Can you work these out from the model? Positions are in its coordinate system, mm. Give positions to 0.01 mm unless a question says otherwise; leave off trailing zeros. Order: outer loops, then holes, each group sorted by start corner. A loop starts at its lowest first (then second) coordinate and runs counter-clockwise, first axis right, second up. Notation, with made-up numbers: M -37,61 L -2,61 A20 ccw -2,94 Z; hole C 65,18.5 d8. An arc over 180 degrees is marked long. Write each question's results on one line, items separated by ' | '.
Solid Edge part; units mm, degrees
sketch "Sketch1" plane through (0, 0, 0) normal (-1, 0, 0) x (0, -1, 0)
  line L0 (0, 20) -> (-5, 20)
  line L1 (-5, 20) -> (-5, 0)
  line L2 (-5, 0) -> (0, 0)
  line L3 (0, 0) -> (0, 20)
extrude "Protrusion1" add sketch "Sketch1" along normal mid plane 90
sketch "Sketch2" plane through (0, 0, 7.5) normal (0, -1, 0) x (1, 0, 0)
  line L0 (-45, 12.5) -> (-50, 12.5)
  line L1 (-50, 12.5) -> (-50, 7.5)
  line L2 (-50, 7.5) -> (-45, 7.5)
  line L3 (-45, 7.5) -> (-45, 12.5)
  line L4 (-45, -2.5) -> (-50, -2.5)
  line L5 (-50, -2.5) -> (-50, -7.5)
  line L6 (-50, -7.5) -> (-45, -7.5)
  line L7 (-45, -7.5) -> (-45, -2.5)
  line L8 (45, 7.5) -> (50, 7.5)
  line L9 (50, 7.5) -> (50, 12.5)
  line L10 (50, 12.5) -> (45, 12.5)
  line L11 (45, 12.5) -> (45, 7.5)
  line L12 (45, -7.5) -> (50, -7.5)
  line L13 (50, -7.5) -> (50, -2.5)
  line L14 (50, -2.5) -> (45, -2.5)
  line L15 (45, -2.5) -> (45, -7.5)
extrude "ExtrudedProtrusion_2" add sketch "Sketch2" against normal blind 5
hole "Hole_1" at (22.5, 0, 10) direction (0, 1, 0) diameter 3 depth 50.8
hole "Hole1" at (-22.5, 0, 10) direction (0, 1, 0) diameter 3 depth 50.8
sketch "Sketch3" plane through (0, 5, 10) normal (0, 1, 0) x (-1, 0, 0)
  line L0 (-50, 10) -> (-45, 10)
  line L1 (-45, 10) -> (-45, -10)
  line L2 (-45, -10) -> (-50, -10)
  line L3 (-50, -10) -> (-50, 10)
  line L4 (50, 10) -> (45, 10)
  line L5 (45, 10) -> (45, -10)
  line L6 (45, -10) -> (50, -10)
  line L7 (50, -10) -> (50, 10)
extrude "ExtrudedCutout_1" cut sketch "Sketch3" against normal blind 5
sketch "Sketch4" plane through (0, 5, 10) normal (0, 1, 0) x (-1, 0, 0)
  line L0 (-50, 10) -> (-45, 10)
  line L1 (-45, 10) -> (-45, -10)
  line L2 (-45, -10) -> (-50, -10)
  line L3 (-50, -10) -> (-50, 10)
  line L4 (45, 10) -> (50, 10)
  line L5 (50, 10) -> (50, -10)
  line L6 (50, -10) -> (45, -10)
  line L7 (45, -10) -> (45, 10)
extrude "ExtrudedProtrusion_3" add sketch "Sketch4" against normal blind 5
hole "Hole_7" at (-45, 0, 15) direction (0, 1, 0) diameter 3.2 end up to next countersink diameter 6.3 countersink angle 90
hole "Hole2" at (-45, 0, 5) direction (0, 1, 0) diameter 3.2 end up to next countersink diameter 6.3 countersink angle 90
hole "Hole3" at (45, 0, 5) direction (0, 1, 0) diameter 3.2 end up to next countersink diameter 6.3 countersink angle 90
hole "Hole4" at (45, 0, 15) direction (0, 1, 0) diameter 3.2 end up to next countersink diameter 6.3 countersink angle 90
hole "Hole_11" at (22.5, 5, 10) direction (0, -1, 0) diameter 3.2 end up to next countersink diameter 6.3 countersink angle 90
hole "Hole5" at (-22.5, 5, 10) direction (0, -1, 0) diameter 3.2 end up to next countersink diameter 6.3 countersink angle 90
fillet "Round_1" radius 1 4 edges at (50, 2.5, 20) (50, 2.5, 0) (-50, 2.5, 20) (-50, 2.5, 0)
properties material "Polycarbonate"
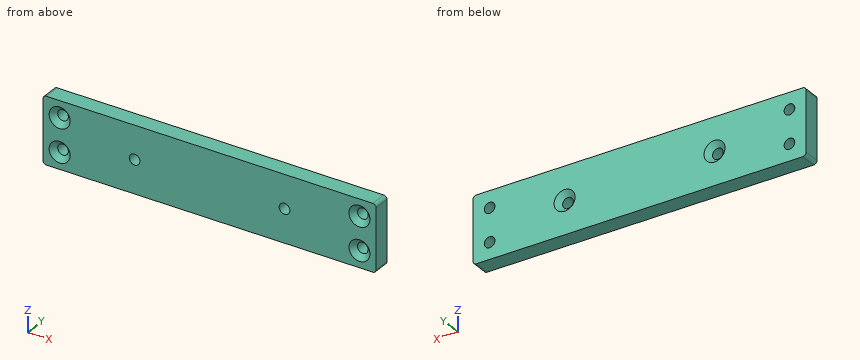
(1) Will this pin go through, and if not, where does the flat tip stop? P1, Ø4, axis at x = 45, z = 15, coming from the -Y side.
Data:
P1: stops at y = 1.15
(2) I need wall thicknesses on L1, parallel to X at y = 1.65, z = 10; L2, parallel to Z at x = -45, y = 3.9; L3, parallel to X at y = 3.9, z = 4.75. Which ranges of each line are inside material? Lowest first, please. Write a range as from..to.
Data:
L1: x = -50..-24.1, -20.9..20.9, 24.1..50 | L2: z = 0..3.4, 6.6..13.4, 16.6..20 | L3: x = -50..-46.58, -43.42..43.42, 46.58..50
(3) Imagine slicing it at B-B, the plane z = 15. Write out the boundary of the cut face in (x, y).
Data:
outline: M -50,0 L -48.15,0 L -46.6,1.55 L -46.6,5 L -50,5 Z; M -43.4,1.55 L -41.85,0 L 41.85,0 L 43.4,1.55 L 43.4,5 L -43.4,5 Z; M 46.6,1.55 L 48.15,0 L 50,0 L 50,5 L 46.6,5 Z
(4) Imagine slicing it at A-A, the plane x = -45. Write out the boundary of the cut face in (y, z).
Data:
outline: M 0,0 L 5,0 L 5,3.4 L 1.55,3.4 L 0,1.85 Z; M 0,8.15 L 1.55,6.6 L 5,6.6 L 5,13.4 L 1.55,13.4 L 0,11.85 Z; M 0,18.15 L 1.55,16.6 L 5,16.6 L 5,20 L 0,20 Z
(5) Imagine slicing it at C-C, the plane x = 22.5. Write out the boundary of the cut face in (y, z), plus the area to 3 significant figures.
Data:
outline: M 0,0 L 5,0 L 5,6.85 L 3.45,8.4 L 0,8.4 Z; M 0,11.6 L 3.45,11.6 L 5,13.15 L 5,20 L 0,20 Z | area: 81.6 mm2
